Source: CAD feature listing. Evaluate the final solid. Frame: model axes, mm. Face numbers are marked on the shaded views. A direction names the side the tool comes from. Give positions to 0.01 mm unless a question says otherwise; leave off trailing zeros. Order: outer loops, then holes, each group sorted by start corner. A loop starts at its lowest first (then second) coordinate and runs counter-clockwise, first axis right, second up. Notation, with made-up numbers: (40, 43.25) -> (54, 43.25) arc R28 ccw to (54, 82.25) -> close; hole circle Ø1 at (-20, 24). An arc over 180 degrees is marked (long way). Answer in a Markdown table with one row per item.
```python
from build123d import *

# Parameters (mm, degrees)
BOSS_EXTRU_1_DEPTH      = 23.5
BOSS_EXTRU_1_DEPTH_BACK = 23.5
CONG_1_R                = 0.5


with BuildPart() as part:
    # Esquisse1 → Boss.-Extru.1 (new, two sides: drawn at the far end of the back side and taken through both)
    with BuildSketch(Plane.ZY.offset(-BOSS_EXTRU_1_DEPTH_BACK)):
        with BuildLine():
            Line((-3.091898803, -3.292916778), (4.377181629, -9.176129997))
            Line((4.377181629, -9.176129997), (6.792591777, -8.531309234))
            Line((6.792591777, -8.531309234), (8.398220531, -6.615074305))
            Line((8.398220531, -6.615074305), (0, 0))
            Line((0, 0), (0.37642312, 3.982248816))
            Line((0.37642312, 3.982248816), (-1.512852543, 4.160833097))
            Line((-1.512852543, 4.160833097), (-3.375381898, 1.938000579))
            ThreePointArc((-3.375381898, 1.938000579), (-17.997095622, 3.097535614), (-12.105520327, 16.529898559))
            Line((-12.105520327, 16.529898559), (1.836440879, 19.428042878))
            Line((1.836440879, 19.428042878), (2.244776367, 23.747898452))
            Line((2.244776367, 23.747898452), (-12.949388907, 20.589455882))
            ThreePointArc((-12.949388907, 20.589455882), (-22.425731532, 2.702545011), (-3.091898803, -3.292916778))
        make_face()
    extrude(amount=BOSS_EXTRU_1_DEPTH + BOSS_EXTRU_1_DEPTH_BACK)

    # Esquisse2 → Fraisage pour vis à tête fraisée M31 (revolve, cut)
    with BuildSketch(Plane(origin=(-13.5, -6.669151695, 1.19442726), x_dir=(0, 0.6187737902502314, -0.7855692181465379), z_dir=(1, 0, 0))):
        Polygon((0, 0), (0, 10.96137699), (1.6, 10), (1.6, 1.7), (2.9, 0.4), (2.9, 0), align=None)
    fraisage_pour_vis_t_te_frais_e_m31 = revolve(axis=Axis((-13.5, -11.657516231, -2.734786308), (0, 0.7855692181465378, 0.6187737902502314)), mode=Mode.SUBTRACT)

    # Symétrie1: Fraisage pour vis à tête fraisée M31 across plane
    add(fraisage_pour_vis_t_te_frais_e_m31.mirror(Plane(origin=(0, 0, 0), x_dir=(0, 0, 1), z_dir=(1, 0, 0))), mode=Mode.SUBTRACT)

    # Congé1
    cong_1_edges = [part.edges().sort_by_distance(p)[0] for p in [
        (-23.5, 22.168677167, -5.35230627),
        (0, -8.531309234, 6.792591777),
        (0, -9.176129997, 4.377181629),
        (0, -3.292916778, -3.091898803),
        (-23.5, 21.587970665, 2.040608623),
        (-23.5, 17.978970719, -5.134539724),
        (-23.5, 3.097535614, -17.997095622),
        (-23.5, 3.049416838, -2.44411722),
        (-23.5, -8.853719615, 5.584886703),
        (-23.5, -6.234523387, 0.642641413),
        (-23.5, 2.702545011, -22.425731532),
        (23.5, 2.702545011, -22.425731532),
        (23.5, 22.168677167, -5.35230627),
        (23.5, 21.587970665, 2.040608623),
        (23.5, 17.978970719, -5.134539724),
        (23.5, 3.097535614, -17.997095622),
        (23.5, 3.049416838, -2.44411722),
        (23.5, -8.853719615, 5.584886703),
        (23.5, -6.234523387, 0.642641413),
    ]]
    fillet(cong_1_edges, radius=CONG_1_R)


solid = part.part
```
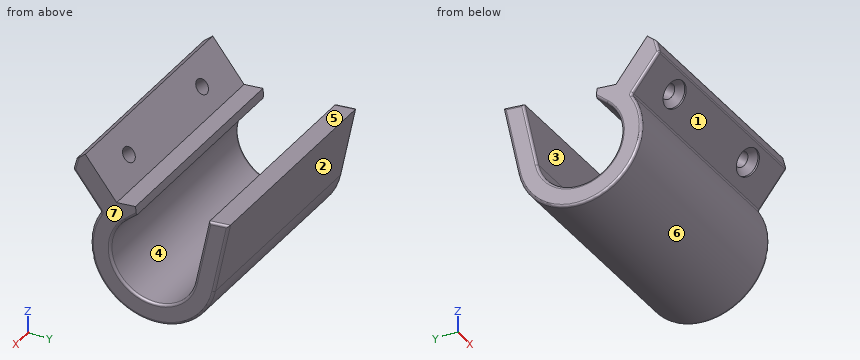
(1) Ray query, probe 1 along Y at (x, z) = (-7.5, -13); probe 2 along Y at (x, z) = (11, -7.5); probe 3 along Z at (x, y) = (20.5, 0.5). Return the intervals inside material, ascending.
A:
| item | result |
|---|---|
| probe 1 | y = -5.14 to -0.86, 16.3 to 20.58 |
| probe 2 | y = -5.13 to -0.84, 17.49 to 21.72 |
| probe 3 | z = -21.26 to -15.65, -4.9 to 0.05 |
(2) Pull-direction query (Y, two-part tool) for the marked faces 4, 5, 6 and 7; classes: +Y half, -Y half, draft (parallel to the pull), parting line (faces both ways), or undercut.
A:
| item | result |
|---|---|
| face 4 | undercut |
| face 5 | undercut |
| face 6 | parting line |
| face 7 | draft |
(3) Section query A-A (x = 2). Return the cut outline in (y, z).
A:
| item | result |
|---|---|
| outline | (-9.11, 4.62) arc R0.5 ccw to (-9.02, 4.18) -> (-3.51, -2.81) arc R0.5 cw to (-3.48, -3.39) arc R13.15 ccw (long way) to (20.59, -12.95) -> (23.75, 2.24) -> (19.43, 1.84) -> (16.53, -12.11) arc R9 cw (long way) to (1.94, -3.38) -> (4.16, -1.51) -> (3.98, 0.38) -> (0, 0) -> (-6.62, 8.4) -> (-8.41, 6.89) arc R0.5 ccw to (-8.57, 6.64) -> close |
(4) Access query for the marked faces 1, 2 and 3. Directions: +Z, -Z, +X, -X, +Y, -Y. A direction counts if a zero-diameter tool reaches every point of the face in a straight line with its end or side. Return the directions, or none.
A:
| item | result |
|---|---|
| face 1 | +X, -X, -Y |
| face 2 | -Z, +X, -X, +Y |
| face 3 | +Z, +X, -X |
(5) First-contact query: pin 1 Ø10 at (x, z) = (6, 2) entering from +Y; pin 2 Ø6 at (x, y) = (9, 3.5) entering from +Z; pin 3 Ø2 at (x, z) = (14, -7.5) entering from +Y. Flat tips, straight axial feed; report the tip coordinate or a pass-through.
A:
| item | result |
|---|---|
| pin 1 | stops at y = 23.75 |
| pin 2 | stops at z = 0.38 |
| pin 3 | stops at y = 21.93 |
